Build history of the part. All positions in model axes, mm. A direction names the side the tool comes from. Give positions to 0.01 mm unless a question says otherwise; leave off trailing zeros. Order: outer loops, then holes, each group sorted by start corner. A loop starts at its lowest first (then second) coordinate and runs counter-clockwise, first axis right, second up. Notation, with made-up numbers: (-9, 8) - (-5, 8) arc R23 cw to (-5, 20) - close; hole circle Ø7 at (-27.75, 15). An arc over 180 degrees is marked (long way). Use a Markdown table: item, result.
from build123d import *

# Parameters (mm, degrees)
F0_W     = 100.4
F0_H     = 81.6
F1_DEPTH = 1
F2_W     = 91.4
F2_H     = 71.6
F3_DEPTH = 5
F4_R     = 5.91518
F5_DEPTH = 25.4


with BuildPart() as f1:
    # F0 (on Top) → F1 (new body)
    with BuildSketch(Plane.XY):
        with Locations((3.041083, 3.351103)):
            Rectangle(F0_W, F0_H)
    extrude(amount=-F1_DEPTH)

    # F2 (on Top) → F3 (join)
    with BuildSketch(Plane.XY):
        with Locations((1.90348, 1.857489)):
            Rectangle(F2_W, F2_H)
    extrude(amount=F3_DEPTH)

    # F4 (on Top) → F5 (cut)
    with BuildSketch(Plane.XY):
        with Locations((0, 44.399735)):
            Circle(F4_R)
    extrude(amount=-F5_DEPTH, mode=Mode.SUBTRACT)


solid = f1.part
1) Slice it at B-B (y = -17). Write the cut outline in (x, z), and give its area (3 significant figures).
Computed:
| item | result |
|---|---|
| outline | (-47.16, -1) - (53.24, -1) - (53.24, 0) - (47.6, 0) - (47.6, 5) - (-43.8, 5) - (-43.8, 0) - (-47.16, 0) - close |
| area | 557 mm² |
2) Pin check, flat tips, straight feed: P1, Ø1.5, axis at y = 13, z = 3, coming from the -X side; P2, Ø1.5, axis at y = -4.5, z = 2.5, coming from the +X side; P3, Ø2.5, axis at x = 6, z = 3.5, coming from the -Y side. Stop position of each tip, or through.
Computed:
| item | result |
|---|---|
| P1 | stops at x = -43.8 |
| P2 | stops at x = 47.6 |
| P3 | stops at y = -33.94 |
3) Wall check: line 1 (Y direction, x = 39, z = 3.6); line 2 (X direction, y = -30, z = 0.8); line 3 (Z direction, x = -27, y = 40). Give the ranges that are in metal, low to high. Write a range as from..to.
Computed:
| item | result |
|---|---|
| line 1 | y = -33.94..37.66 |
| line 2 | x = -43.8..47.6 |
| line 3 | z = -1..0 |
4) Slice it at A-A (x = 0). Write the cut outline in (y, z), and give its area (3 significant figures).
Computed:
| item | result |
|---|---|
| outline | (-37.45, -1) - (38.48, -1) - (38.48, 0) - (37.66, 0) - (37.66, 5) - (-33.94, 5) - (-33.94, 0) - (-37.45, 0) - close |
| area | 434 mm² |
5) Tool access for faces 1 (the flat face through (1, 37.657, 2)), 2 (the flat face through (1, 2, 5)), 3 (the flat face through (1, -33.943, 2)): list every direction of +Z, -Z, +X, -X, +Y, -Y with a clear straight run to the whole face (end or side of a thin tool).
Computed:
| item | result |
|---|---|
| face 1 | +Z, +X, -X, +Y |
| face 2 | +Z, +X, -X, +Y, -Y |
| face 3 | +Z, +X, -X, -Y |
6) Two-plate mould, pull along X, no slides. Class faces 4 (the flat face through (-43.797, 1, 2)), 5 (the flat face through (47.603, 1, 2)), 6 (the cylindrical face through (-0.127, 38.486, -0.493)): +X half, -X half, draft (parallel to the pull), parting line (faces both ways), or undercut.
Computed:
| item | result |
|---|---|
| face 4 | -X half |
| face 5 | +X half |
| face 6 | undercut |
7) Slice it at C-C (z = 1.45). Write the cut outline in (x, y), and give its area (3 significant figures).
Computed:
| item | result |
|---|---|
| outline | (-43.8, -33.94) - (47.6, -33.94) - (47.6, 37.66) - (-43.8, 37.66) - close |
| area | 6,540 mm² |
